from build123d import *

# Parameters (mm, degrees)
SKETCH1_R           = 2.25
SKETCH1_R_2         = 2.5
BOSS_EXTRUDE1_DEPTH = 7
CUT_EXTRUDE1_DEPTH  = 4
CUT_EXTRUDE2_DEPTH  = 4
CUT_EXTRUDE3_DEPTH  = 4


with BuildPart() as part:
    # Sketch1 → Boss-Extrude1 (new body)
    with BuildSketch(Plane(origin=(0, 0, 0), x_dir=(1, 0, 0), z_dir=(0, 1, 0))):
        with BuildLine():
            Line((-35, 48), (-35, -46.101))
            ThreePointArc((-35, -46.101), (-34.553630735, -47.178630735), (-33.476, -47.625))
            Line((-33.476, -47.625), (-23.824, -47.625))
            ThreePointArc((-23.824, -47.625), (-22.746369265, -47.178630735), (-22.3, -46.101))
            Line((-22.3, -46.101), (-22.3, -38.924))
            ThreePointArc((-22.3, -38.924), (-21.853630735, -37.846369265), (-20.776, -37.4))
            Line((-20.776, -37.4), (20.776, -37.4))
            ThreePointArc((20.776, -37.4), (21.853630735, -37.846369265), (22.3, -38.924))
            Line((22.3, -38.924), (22.3, -46.101))
            ThreePointArc((22.3, -46.101), (22.746369265, -47.178630735), (23.824, -47.625))
            Line((23.824, -47.625), (33.476, -47.625))
            ThreePointArc((33.476, -47.625), (34.553630735, -47.178630735), (35, -46.101))
            Line((35, -46.101), (35, 48))
            ThreePointArc((35, 48), (32.803300859, 53.303300859), (27.5, 55.5))
            Line((27.5, 55.5), (18, 55.5))
            ThreePointArc((18, 55.5), (12.696699141, 53.303300859), (10.5, 48))
            Line((10.5, 48), (10.5, 38.924))
            ThreePointArc((10.5, 38.924), (10.053630735, 37.846369265), (8.976, 37.4))
            Line((8.976, 37.4), (-8.976, 37.4))
            ThreePointArc((-8.976, 37.4), (-10.053630735, 37.846369265), (-10.5, 38.924))
            Line((-10.5, 38.924), (-10.5, 48))
            ThreePointArc((-10.5, 48), (-12.696699141, 53.303300859), (-18, 55.5))
            Line((-18, 55.5), (-27.5, 55.5))
            ThreePointArc((-27.5, 55.5), (-32.803300859, 53.303300859), (-35, 48))
        make_face()
        with Locations(Location((-18, 48, 0), (0, 0, 270))):  # turned: the seam where the file's is
            Circle(SKETCH1_R, mode=Mode.SUBTRACT)
        with Locations(Location((18, 48, 0), (0, 0, 270))):  # turned: the seam where the file's is
            Circle(SKETCH1_R, mode=Mode.SUBTRACT)
        with Locations(Location((-18, 30, 0), (0, 0, 270))):  # turned: the seam where the file's is
            Circle(SKETCH1_R, mode=Mode.SUBTRACT)
        with Locations(Location((18, 30, 0), (0, 0, 270))):  # turned: the seam where the file's is
            Circle(SKETCH1_R, mode=Mode.SUBTRACT)
        with Locations(Location((-29.5, 42, 0), (0, 0, 270))):  # turned: the seam where the file's is
            Circle(SKETCH1_R, mode=Mode.SUBTRACT)
        with Locations(Location((-29.5, 8, 0), (0, 0, 270))):  # turned: the seam where the file's is
            Circle(SKETCH1_R, mode=Mode.SUBTRACT)
        with Locations(Location((-29.5, -8, 0), (0, 0, 270))):  # turned: the seam where the file's is
            Circle(SKETCH1_R, mode=Mode.SUBTRACT)
        with Locations(Location((-29.5, -42, 0), (0, 0, 270))):  # turned: the seam where the file's is
            Circle(SKETCH1_R, mode=Mode.SUBTRACT)
        with Locations(Location((29.5, -8, 0), (0, 0, 270))):  # turned: the seam where the file's is
            Circle(SKETCH1_R, mode=Mode.SUBTRACT)
        with Locations(Location((29.5, -42, 0), (0, 0, 270))):  # turned: the seam where the file's is
            Circle(SKETCH1_R, mode=Mode.SUBTRACT)
        with Locations(Location((29.5, 42, 0), (0, 0, 270))):  # turned: the seam where the file's is
            Circle(SKETCH1_R, mode=Mode.SUBTRACT)
        with Locations(Location((29.5, 8, 0), (0, 0, 270))):  # turned: the seam where the file's is
            Circle(SKETCH1_R, mode=Mode.SUBTRACT)
        with Locations(Location((-25, 0, 0), (0, 0, 270))):  # turned: the seam where the file's is
            Circle(SKETCH1_R_2, mode=Mode.SUBTRACT)
        with Locations(Location((25, 0, 0), (0, 0, 270))):  # turned: the seam where the file's is
            Circle(SKETCH1_R_2, mode=Mode.SUBTRACT)
        with BuildLine():
            Line((-9, -19.14172824), (-9, -23.876))
            ThreePointArc((-9, -23.876), (-8.553630735, -24.953630735), (-7.476, -25.4))
            Line((-7.476, -25.4), (7.476, -25.4))
            ThreePointArc((7.476, -25.4), (8.553630735, -24.953630735), (9, -23.876))
            Line((9, -23.876), (9, -19.14172824))
            ThreePointArc((9, -19.14172824), (9.212217545, -18.365968747), (9.789767442, -17.806258828))
            ThreePointArc((9.789767442, -17.806258828), (20.32, 0), (9.789767442, 17.806258828))
            ThreePointArc((9.789767442, 17.806258828), (9.212217545, 18.365968747), (9, 19.14172824))
            Line((9, 19.14172824), (9, 23.876))
            ThreePointArc((9, 23.876), (8.553630735, 24.953630735), (7.476, 25.4))
            Line((7.476, 25.4), (-7.476, 25.4))
            ThreePointArc((-7.476, 25.4), (-8.553630735, 24.953630735), (-9, 23.876))
            Line((-9, 23.876), (-9, 19.14172824))
            ThreePointArc((-9, 19.14172824), (-9.212217545, 18.365968747), (-9.789767442, 17.806258828))
            ThreePointArc((-9.789767442, 17.806258828), (-20.32, 0), (-9.789767442, -17.806258828))
            ThreePointArc((-9.789767442, -17.806258828), (-9.212217545, -18.365968747), (-9, -19.14172824))
        make_face(mode=Mode.SUBTRACT)
    extrude(amount=BOSS_EXTRUDE1_DEPTH)

    # Sketch2 → Cut-Extrude1 (cut)
    with BuildSketch(Plane(origin=(0, 7, 0), x_dir=(1, 0, 0), z_dir=(0, 1, 0))):
        Polygon((-26.324573519, 42), (-27.91228676, 44.75), (-31.08771324, 44.75), (-32.675426481, 42), (-31.08771324, 39.25), (-27.91228676, 39.25), align=None)
        Polygon((26.324573519, 42), (27.91228676, 39.25), (31.08771324, 39.25), (32.675426481, 42), (31.08771324, 44.75), (27.91228676, 44.75), align=None)
        Polygon((26.324573519, 8), (27.91228676, 5.25), (31.08771324, 5.25), (32.675426481, 8), (31.08771324, 10.75), (27.91228676, 10.75), align=None)
        Polygon((26.324573519, -8), (27.91228676, -10.75), (31.08771324, -10.75), (32.675426481, -8), (31.08771324, -5.25), (27.91228676, -5.25), align=None)
        Polygon((26.324573519, -42), (27.91228676, -44.75), (31.08771324, -44.75), (32.675426481, -42), (31.08771324, -39.25), (27.91228676, -39.25), align=None)
        Polygon((-26.324573519, -42), (-27.91228676, -39.25), (-31.08771324, -39.25), (-32.675426481, -42), (-31.08771324, -44.75), (-27.91228676, -44.75), align=None)
        Polygon((-26.324573519, -8), (-27.91228676, -5.25), (-31.08771324, -5.25), (-32.675426481, -8), (-31.08771324, -10.75), (-27.91228676, -10.75), align=None)
        Polygon((-26.324573519, 8), (-27.91228676, 10.75), (-31.08771324, 10.75), (-32.675426481, 8), (-31.08771324, 5.25), (-27.91228676, 5.25), align=None)
    extrude(amount=-CUT_EXTRUDE1_DEPTH, mode=Mode.SUBTRACT)

    # Sketch3 → Cut-Extrude2 (cut)
    with BuildSketch(Plane.XZ):
        Polygon((-18, -33.175426481), (-15.25, -31.58771324), (-15.25, -28.41228676), (-18, -26.824573519), (-20.75, -28.41228676), (-20.75, -31.58771324), align=None)
        Polygon((-18, -51.175426481), (-15.25, -49.58771324), (-15.25, -46.41228676), (-18, -44.824573519), (-20.75, -46.41228676), (-20.75, -49.58771324), align=None)
        Polygon((18, -51.175426481), (20.75, -49.58771324), (20.75, -46.41228676), (18, -44.824573519), (15.25, -46.41228676), (15.25, -49.58771324), align=None)
        Polygon((18, -33.175426481), (20.75, -31.58771324), (20.75, -28.41228676), (18, -26.824573519), (15.25, -28.41228676), (15.25, -31.58771324), align=None)
    extrude(amount=-CUT_EXTRUDE2_DEPTH, mode=Mode.SUBTRACT)

    # Sketch4 → Cut-Extrude3 (cut)
    with BuildSketch(Plane.XZ):
        Polygon((-25, -4.330127019), (-21.25, -2.165063509), (-21.25, 2.165063509), (-25, 4.330127019), (-28.75, 2.165063509), (-28.75, -2.165063509), align=None)
        Polygon((25, -4.330127019), (28.75, -2.165063509), (28.75, 2.165063509), (25, 4.330127019), (21.25, 2.165063509), (21.25, -2.165063509), align=None)
    extrude(amount=-CUT_EXTRUDE3_DEPTH, mode=Mode.SUBTRACT)


solid = part.part
CAD build for the part. Positions are in the model's coordinates, mm. A direction names the side the tool comes from. Give positions to 0.01 mm unless a question says otherwise; leave off trailing zeros. Write each loop counter-clockwise with the first axis right and the second up, starting at its lowest first coordinate (ties: lowest second). Pieces come first, ordered by that corner, then holes. Notation, with made-up numbers: (-30.5, 77.25) - (-11.5, 77.25) arc R25 cw to (-11.5, 112.25) - close; hole circle Ø7 at (80, 44.5). An arc over 180 degrees is marked (long way). Put each result on its own line as item: value.
(1) Pull direction Z, two halves, no side cores. Call faces 1 (the flat face through (-29, 3, 47.625)), 2 (the cylindrical face through (-12.639, 3.451, -53.245)), 3 (the flat face through (-31.89, 5.03, -6.64)): released by +Z, released by -Z, zero draft, split by the parting line, or undercut.
Working result:
face 1: released by +Z
face 2: released by -Z
face 3: undercut
(2) Saw through at A-A (z = -30). List the corners of the cut face in (x, y), then the cut area to 3 significant figures.
Working result:
outline: (-35, 0) - (-20.75, 0) - (-20.75, 4) - (-20.25, 4) - (-20.25, 7) - (-35, 7) - close; (-15.75, 4) - (-15.25, 4) - (-15.25, 0) - (15.25, 0) - (15.25, 4) - (15.75, 4) - (15.75, 7) - (-15.75, 7) - close; (20.25, 4) - (20.75, 4) - (20.75, 0) - (35, 0) - (35, 7) - (20.25, 7) - close
area: 419 mm^2
(3) Drop flat-ended pins along their axis: pin 1 Ø4 at (x, y) = (-8.5, 2) entering from +Z; pin 2 Ø4.5 at (x, z) = (-25, 0) entering from -Y; pin 3 Ø1 at (x, y) = (29.5, 5.5) entering from -Z; pin 4 Ø4.5 at (x, z) = (17, -29) entering from -Y. Give the stop position or say it passes through.
Working result:
pin 1: z = 37.4
pin 2: through
pin 3: z = -55.35
pin 4: y = 0
(4) Wall check: L1, parallel to X at y = 1.9, z = -42; L2, parallel to X at y = 6.1, z = -30; L3, parallel to X at y = 0.9, z = 42. Give the ranges that are in metal, low to high.
Working result:
L1: -35 to -31.75, -27.25 to -10.5, 10.5 to 27.25, 31.75 to 35
L2: -35 to -20.25, -15.75 to 15.75, 20.25 to 35
L3: -35 to -31.75, -27.25 to -22.3, 22.3 to 27.25, 31.75 to 35
(5) Saw through at D-D (y = 6). Count the separate pieces of the cut face and the enclosed holes in it, then the cut area to 3 significant figures.
Working result:
separate pieces: 1
enclosed holes: 15
area: 4,520 mm^2
(6) Saw through at C-C (z = 7). List the corners of the cut face in (x, y), then the cut area to 3 significant figures.
Working result:
outline: (-35, 0) - (-31.52, 0) - (-31.52, 3) - (-32.1, 3) - (-32.1, 7) - (-35, 7) - close; (-27.48, 0) - (-19.08, 0) - (-19.08, 7) - (-26.9, 7) - (-26.9, 3) - (-27.48, 3) - close; (19.08, 0) - (27.48, 0) - (27.48, 3) - (26.9, 3) - (26.9, 7) - (19.08, 7) - close; (31.52, 0) - (35, 0) - (35, 7) - (32.1, 7) - (32.1, 3) - (31.52, 3) - close
area: 157 mm^2
(7) Tool access for faces 4 (the flat face through (16.606, 1.972, -50.37)), 5 (the flat face through (31.89, 5.03, -43.36)): list every direction of +Z, -Z, +X, -X, +Y, -Y with a clear straight run to the whole face (end or side of a thin tool).
Working result:
face 4: -Y
face 5: +Y
(8) Saw through at B-B (x = 1.5). List the corners of the cut face in (y, z).
Working result:
outline: (0, -37.4) - (7, -37.4) - (7, -25.4) - (0, -25.4) - close; (0, 25.4) - (7, 25.4) - (7, 37.4) - (0, 37.4) - close
